Job drawing, mm, ordinate dimensions from the low corner. One solid piece. Round coordinates to 2 decimals unless told otherwise and drop trailing zeros. Write each loop counter-clockwise with the first axis right and the second up, starting at its lowest first coordinate (ties: lowest second). Pieces come first, ordered by that corner, then holes.
1) Saw through at B-B on z = 26. Write the cut outline in (x, y).
2) Saw through at A-A on y = 22. Write the cut outline in (x, z), and give its area (3 significant figures).
3) Drill centre lines: L1, parallel to Y at x = 31.5, z = 20; L2, parallel to X at y = 12, z = 6.5; L3, parallel to Y at x = 22, z = 15.5. Where is each one in solid material? Low to high.
4) Flat gauge pins, fed straight in: pin 1 (12 mm diameter, centred on x = 28.5, z = 11.5, fed in from +Y); pin 2 (1 mm diameter, centred on x = 8.5, y = 23.5, fed in from -Z); pin 3 (1.5 mm diameter, centred on x = 10, y = 33.5, fed in from +Z). Where does each tip first touch, or does it go through?
5) Pull direction Y, two halves, no side cores. Call the marked faces 1, 2 and 3: +Y half, -Y half, draft (parallel to the pull), parting line (faces both ways), or undercut.
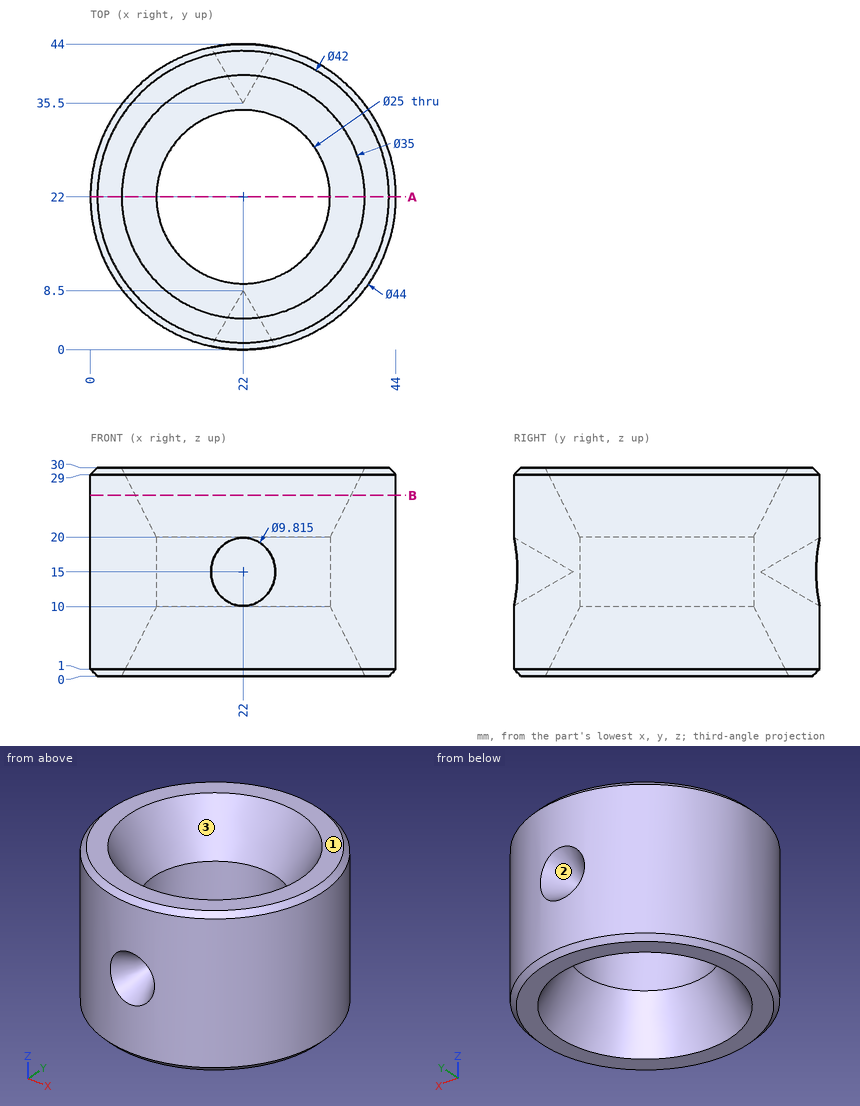
Completed:
1. outline: circle Ø44 at (22, 22); hole circle Ø31 at (22, 22)
2. outline: (0, 1) - (1, 0) - (4.5, 0) - (9.5, 10) - (9.5, 20) - (4.5, 30) - (1, 30) - (0, 29) - close; (34.5, 10) - (39.5, 0) - (43, 0) - (44, 1) - (44, 29) - (43, 30) - (39.5, 30) - (34.5, 20) - close
2. area: 468 mm2
3. L1: y = 2.16 to 13.88, 30.12 to 41.84
3. L2: x = 2.4 to 11.85, 32.15 to 41.6
3. L3: y = 7.63 to 9.5, 34.5 to 36.37
4. pin 1: stops at y = 43.99
4. pin 2: stops at z = 6.83
4. pin 3: stops at z = 29.74
5. face 1: draft
5. face 2: +Y half
5. face 3: undercut
